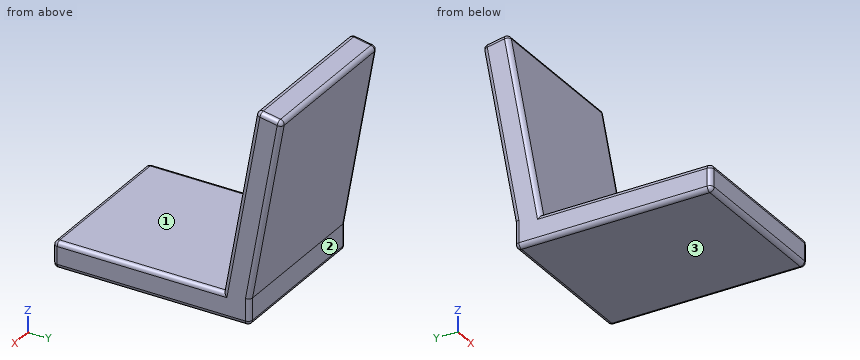
from build123d import *

# Parameters (mm, degrees)
F0_W     = 360
F0_H     = 450
F1_DEPTH = 60
F3_DEPTH = 360
F4_R     = 10


with BuildPart() as f1:
    # F0 (on Top) → F1 (new body)
    with BuildSketch(Plane.XY):
        Rectangle(F0_W, F0_H)
    extrude(amount=F1_DEPTH)

    # F2 (on face) → F3 (join, through all)
    with BuildSketch(Plane(origin=(-180, 0, 0), x_dir=(0, -1, 0), z_dir=(-1, 0, 0))):
        Polygon((-298.98347, 479.581109), (-225, 60), (-164.074403, 60), (-239.895005, 490), align=None)
    extrude(amount=-F3_DEPTH)

    # F4
    f4_edges = [f1.edges().sort_by_distance(p)[0] for p in [
        (-180, 225, 30),
        (-180, 261.991735, 269.790555),
        (-180, 269.439238, 484.790555),
        (-180, 201.984704, 275),
        (-180, -30.462798, 60),
        (-180, -225, 30),
        (-180, 0, 0),
        (180, -225, 30),
        (180, -30.462798, 60),
        (180, 201.984704, 275),
        (180, 269.439238, 484.790555),
        (180, 261.991735, 269.790555),
        (180, 225, 30),
        (180, 0, 0),
        (0, -225, 0),
        (0, -225, 60),
        (0, 239.895005, 490),
        (0, 298.98347, 479.581109),
        (0, 225, 0),
    ]]
    fillet(f4_edges, radius=F4_R)


solid = f1.part
Part model, mm, in its own coordinate system. Face numbers are marked on the shaded views. A direction names the side the tool comes from. Coordinates: 2 decimals unless noted, no trailing zeros. Order: outer loops, then holes, each group sorted by start corner. A loop starts at its lowest first (then second) coordinate and runs counter-clockwise, first axis right, second up. Notation, with made-up numbers: M 36.5,-1 L 63.5,-1 A4 cw 63.5,3 Z; hole C -34,8 d11. An arc over 180 degrees is marked long. Use a Markdown table: item, result.
(1) Cut at A-A on x = 125.5. Write the cut outline in (y, z).
A:
| item | result |
|---|---|
| outline | M -225,10 A10 ccw -215,0 L 215,0 A10 ccw 225,10 L 225,60 L 297.25,469.73 A10 ccw 289.14,481.32 L 249.74,488.26 A10 ccw 238.16,480.15 L 164.07,60 L -215,60 A10 ccw -225,50 Z |
(2) Flat gauge pins, fed straight in: pin 1 (3 mm diameter, centred on x = -71.5, z = 274.5, fed in from -Y); pin 2 (12 mm diameter, centred on x = 28.5, z = 393, fed in from +Y); pin 3 (6 mm diameter, centred on x = 127, z = 387, fed in from +Y); pin 4 (1.5 mm diameter, centred on x = 74, y = -148.5, fed in from -Z). Where does each tip first touch, or does it go through?
A:
| item | result |
|---|---|
| pin 1 | stops at y = 201.63 |
| pin 2 | stops at y = 284.77 |
| pin 3 | stops at y = 283.19 |
| pin 4 | stops at z = 0 |
(3) Cut at C-C on y = 125. Write the cut outline in (x, z).
A:
| item | result |
|---|---|
| outline | M -180,10 A10 ccw -170,0 L 170,0 A10 ccw 180,10 L 180,50 A10 ccw 170,60 L -170,60 A10 ccw -180,50 Z |
(4) Tool access for the marked faces 1, 2 and 3: list every direction of +Z, -Z, +X, -X, +Y, -Y with a clear straight run to the whole face (end or side of a thin tool).
A:
| item | result |
|---|---|
| face 1 | +Z, +X, -X, -Y |
| face 2 | -Z, +X, -X, +Y |
| face 3 | -Z, +X, -X, +Y, -Y |
(5) Cut at B-B on z = 34.5. Write the cut outline in (x, y), then the cut area to 3 significant figures.
A:
| item | result |
|---|---|
| outline | M -180,-215 A10 ccw -170,-225 L 170,-225 A10 ccw 180,-215 L 180,215 A10 ccw 170,225 L -170,225 A10 ccw -180,215 Z |
| area | 162,000 mm^2 |
(6) Probe L1, parallel to Z at x = 98, y = -125; L2, parallel to Y at x = -33, z = 36; L3, parallel to X at y = 206, z = 243.5. List the from-to ranges inside material, lowest first.
A:
| item | result |
|---|---|
| L1 | z = 0 to 60 |
| L2 | y = -225 to 225 |
| L3 | x = -179.98 to 179.98 |
